```python
from build123d import *

# Parameters (mm, degrees)
SKETCH1_W           = 60
SKETCH1_H           = 9.5
BOSS_EXTRUDE1_DEPTH = 9.5
SKETCH4_W           = 11.588990026
SKETCH4_H           = 9.5
BOSS_EXTRUDE2_DEPTH = 24
SKETCH1_2_W         = 60
SKETCH1_2_H         = 9.5
BOSS_EXTRUDE3_DEPTH = 10
SKETCH7_R           = 3.1
CUT_EXTRUDE2_DEPTH  = 38.921447552
BOSS_EXTRUDE7_DEPTH = 9.5
CHAMFER1_SIZE       = 1
CHAMFER1_SIZE2      = 0.554309051


with BuildPart() as part:
    # Sketch1 → Boss-Extrude1 (new body)
    with BuildSketch(Plane(origin=(0, 0, 0), x_dir=(1, 0, 0), z_dir=(0, 1, 0))):
        with Locations((30, 4.75)):
            Rectangle(SKETCH1_W, SKETCH1_H)
    extrude(amount=BOSS_EXTRUDE1_DEPTH)

    # Sketch4 → Boss-Extrude2 (add)
    with BuildSketch(Plane(origin=(-2.375, 8.863620668, 0), x_dir=(0.965925826, 0.258819045, 0), z_dir=(-0.258819045, 0.965925826, 0))):
        with Locations((8.253275941, 4.75)):
            Rectangle(SKETCH4_W, SKETCH4_H)
    extrude(amount=-BOSS_EXTRUDE2_DEPTH)

    # Sketch1_2 → Boss-Extrude3 (add)
    with BuildSketch(Plane(origin=(0, 0, 0), x_dir=(1, 0, 0), z_dir=(0, 1, 0))):
        with Locations((30, 4.75)):
            Rectangle(SKETCH1_2_W, SKETCH1_2_H)
    extrude(amount=-BOSS_EXTRUDE3_DEPTH)

    # Sketch7 → Cut-Extrude2 (cut, through all)
    with BuildSketch(Plane(origin=(-2.375, 8.863620668, 0), x_dir=(0.965925826, 0.258819045, 0), z_dir=(-0.258819045, 0.965925826, 0))):
        with Locations((8, 4.75)):
            Circle(SKETCH7_R)
    extrude(amount=-CUT_EXTRUDE2_DEPTH, mode=Mode.SUBTRACT)

    # Sketch13 → Boss-Extrude7 (add)
    with BuildSketch(Plane(origin=(0, 0, -9.5), x_dir=(-1, 0, 0), z_dir=(0, 0, -1))):
        Polygon((-6.211657082, -13.682219831), (0, -10), (-5.225009252, -10), align=None)
    extrude(amount=-BOSS_EXTRUDE7_DEPTH)

    # Chamfer1
    chamfer1_edges = [part.edges().sort_by_distance(p)[0] for p in [
        (60, 9.5, -4.75),
        (60, -10, -4.75),
        (60, -0.25, -9.5),
        (60, -0.25, 0),
    ]]
    chamfer1_side = [part.faces().sort_by_distance(p)[0] for p in [
        (60, -0.25, -4.75),
    ]]
    chamfer(chamfer1_edges, length=CHAMFER1_SIZE, length2=CHAMFER1_SIZE2, reference=chamfer1_side[0])


solid = part.part
```
For this review, take the finished solid that the model builds, in its own axes (mm). A direction names the side the tool comes from. Round coordinates to 2 decimals unless told otherwise and drop trailing zeros. Write each loop counter-clockwise with the first axis right and the second up, starting at its lowest first coordinate (ties: lowest second). Pieces come first, ordered by that corner, then holes. Notation, with made-up numbers: (8.5, 83) -> (15.5, 83) arc R11 ccw to (15.5, 103) -> close; hole circle Ø5 at (-37.75, 20). An arc over 180 degrees is marked (long way). One line per question, with ' | ' between items. Start each with the question number.
1) Wall thickness on line 1 along Z through (x, y) = (5.5, 10.5); line 2 along Y through (x, z) = (48, -4); line 3 along Z through (x, y) = (10, -3): over which ranges is each line inside the solid? List them lowest first.
2) Add section B-B (x = 30.5). Write out the cut boundary in (y, z).
3) Mouldability with a two-part tool opening along Z and no side actions: class faces 1 (the flat face through (59.719, 9.007, -4.684)), 2 (the cylindrical face through (7.766, -0.669, -1.724)), 3 (the flat face through (30, 0, -9.5)) as +Z half, -Z half, draft (parallel to the pull), parting line (faces both ways), or undercut.
4) Add section C-C (z = -2.25). Write out the cut boundary in (x, y), and give its area (3 significant figures).
5) For pin 1 Ø5 at (x, z) = (31, -5.5) entering from +Y, flat-tipped, find the tip position at first contact; note if it passes through.
6) Machinability: for faces 4 (the flat face through (60, 0, -5)), 5 (the flat face through (35, 9.5, -5)), which of the approach directions +Z, -Z, +X, -X, +Y, -Y give a long, thin tool a straight path to every point of the face, cutting with its end or side? Answer none if there is none.
7) Add section A-A (z = -5.75). Write out the cut boundary in (x, y), and give its area (3 significant figures).
Reported:
1) line 1: z = -9.5 to -7.85, -1.65 to 0 | line 2: y = -10 to 9.5 | line 3: z = -9.5 to -7.72, -1.78 to 0
2) outline: (-10, -9.5) -> (9.5, -9.5) -> (9.5, 0) -> (-10, 0) -> close
3) face 1: draft | face 2: undercut | face 3: -Z half
4) outline: (0, -10) -> (6.21, -13.68) -> (9.79, -12.72) -> (3.58, 10.46) -> (0, 9.5) -> close; (7.12, 11.41) -> (13.33, -11.77) -> (17.41, -10.68) -> (17.22, -10) -> (59.45, -10) -> (60, -9) -> (60, 8.5) -> (59.45, 9.5) -> (12, 9.5) -> (11.19, 12.5) -> close | area: 1,140 mm²
5) pin 1: stops at y = 9.5
6) face 4: +Z, -Z, +X, +Y, -Y | face 5: +Z, -Z, +X, +Y
7) outline: (0, -10) -> (6.21, -13.68) -> (8.73, -13.01) -> (2.52, 10.17) -> (0, 9.5) -> close; (8.19, 11.69) -> (14.4, -11.49) -> (17.41, -10.68) -> (17.22, -10) -> (59.45, -10) -> (60, -9) -> (60, 8.5) -> (59.45, 9.5) -> (12, 9.5) -> (11.19, 12.5) -> close | area: 1,080 mm²
